Check sheet for the modelled part. Datum: model origin and axes. Units: mm. A direction names the side the tool comes from. Coordinates: 2 decimals unless noted, no trailing zeros. One line per item, written item: value. Start each with the question number.
1) Scan lines: line 1 along Z through (x, y) = (0, 5.5); line 2 along Z through (x, y) = (0.5, -16); line 3 along X through (y, z) = (-14.25, 230). Record each from-to range of solid material in increasing order. Write a range as [from, to].
2) Draft check along X on faces 3 (the cylindrical face through (-0.59, 4.52, -4.46)), 4 (the flat face through (20, 0, 4)), 5 (the flat face through (4, 0, 250)). Enter one of: +X half, -X half, draft (parallel to the pull), parting line (faces both ways), or undercut.
3) Set-up check for faces 1 (the cylindrical face through (7.493, -15.76, -0.33)), 2 (the cylindrical face through (-3.32, 4.52, -233.04)): record each of +Z, -Z, +X, -X, +Y, -Y from which the full face is reachable in a straight line by a thin tool's end or side.
4) Gauge pin test, flat ends, axial feed: P1, Ø5.5, axis at x = 0, z = 0, coming from the -Y side; P2, Ø4.5, axis at x = 0, z = 233.5, coming from the -Y side; P3, Ø5.5, axis at x = 0, y = 0, coming from the -Z side; P4, Ø6, axis at x = 0, y = 0, coming from the -Z side. Record the tip position at first contact, or that the pin passes through.
```python
from build123d import *

# Parameters (mm, degrees)
SKETCH1_W                                           = 40
SKETCH1_H                                           = 40
SKETCH1_R                                           = 2.5
BOSS_EXTRUDE1_DEPTH                                 = 250
FILLET1_R                                           = 2
CBORE_FOR_M8_HEX_SOCKET_HEAD_CAP_SCREW1_D           = 9
CBORE_FOR_M8_HEX_SOCKET_HEAD_CAP_SCREW1_CBORE_D     = 15
CBORE_FOR_M8_HEX_SOCKET_HEAD_CAP_SCREW1_CBORE_DEPTH = 8.6


with BuildPart() as part:
    # Sketch1 → Boss-Extrude1 (new, symmetric)
    with BuildSketch(Plane.XY):
        Rectangle(SKETCH1_W, SKETCH1_H)
        Circle(SKETCH1_R, mode=Mode.SUBTRACT)
    extrude(amount=BOSS_EXTRUDE1_DEPTH, both=True)

    # Fillet1
    fillet1_edges = [part.edges().sort_by_distance(p)[0] for p in [
        (20, -20, 0),
        (-20, -20, 0),
        (-20, 20, 0),
        (20, 20, 0),
    ]]
    fillet(fillet1_edges, radius=FILLET1_R)

    # CBORE for M8 Hex Socket Head Cap Screw1 (through all)
    with Locations(Plane(origin=(0, -20, 0), x_dir=(-1, 0, 0), z_dir=(0, -1, 0))):
        with Locations((0, 500), (0, 0), (0, -500), (0, 230), (0, -230)):
            CounterBoreHole(CBORE_FOR_M8_HEX_SOCKET_HEAD_CAP_SCREW1_D / 2, CBORE_FOR_M8_HEX_SOCKET_HEAD_CAP_SCREW1_CBORE_D / 2, CBORE_FOR_M8_HEX_SOCKET_HEAD_CAP_SCREW1_CBORE_DEPTH)

    # Sketch9 → M8x1.25 Tapped Hole1 (revolve, cut)
    with BuildSketch(Plane(origin=(0, 0, 250), x_dir=(0, -1, 0), z_dir=(1, 0, 0))):
        Polygon((0, 0), (0, 29.792926105), (3.4, 27.75), (3.4, 0), align=None)
    m8x1_25_tapped_hole1 = revolve(axis=Axis((0, 0, 256.35), (0, 0, -1)), mode=Mode.SUBTRACT)

    # Mirror1: M8x1.25 Tapped Hole1 across plane
    add(m8x1_25_tapped_hole1.mirror(Plane.XY), mode=Mode.SUBTRACT)


solid = part.part
```
Answers:
1. line 1: z = [-250, -234.5], [-225.5, -4.5], [4.5, 225.5], [234.5, 250]
1. line 2: z = [-250, -237.48], [-222.52, -7.48], [7.48, 222.52], [237.48, 250]
1. line 3: x = [-20, -7.5], [7.5, 20]
2. face 3: undercut
2. face 4: +X half
2. face 5: draft
3. face 1: -Y
3. face 2: +Y, -Y
4. P1: passes through
4. P2: stops at y = -11.4
4. P3: stops at z = -221.86
4. P4: stops at z = -222.01
